Geometry: final body of the model. Coordinates: model frame, mm. Give positions to 0.01 mm unless a question says otherwise; leave off trailing zeros. Write each loop counter-clockwise with the first axis right and the second up, starting at its lowest first coordinate (ties: lowest second). Pieces come first, ordered by that corner, then holes. Notation, with made-up numbers: M -40,-0.75 L -18,-0.75 A17 cw -18,32.25 Z; hole C 56,-3.5 d7. An arc over 180 degrees is marked long. Use a Markdown table: item, result. Add a question column.
(1) Cut plane B-B (y = 326). Output: boundary loops of the cut face in (x, z) (3 decimals), plus the area to 3 significant figures.
(2) Pin query (flat end, axial travel): pin 1 Ø1 at (y, z) = (349.5, 1) entering from +X; pin 2 Ø1.6 at (x, z) = (287, 1.5) entering from +Y; pin 3 Ø1.6 at (x, z) = (287.5, 1.5) entering from -Y. Return the tip coordinate at first contact, or that it passes through.
(3) Cut plane C-C (x = 226.5). Output: boundary loops of the cut face in (y, z) (3 decimals).
(4) Material intervals for L1, parallel to X at y = -335.5, z = 0.75; L2, parallel to Y at x = 267, z = 1.4; L3, parallel to Y at x = 165, z = 1.85, sorted ascending.
(5) Cut plane A-A (z = 1.1). Output: boundary loops of the cut face in (x, y).
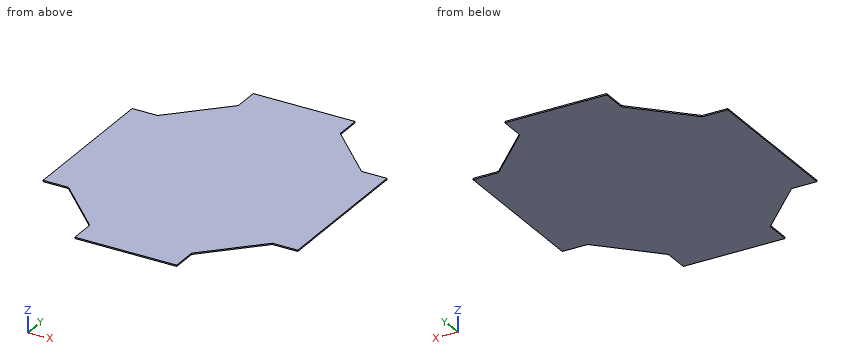
```python
from build123d import *

# Parameters (mm, degrees)
SKETCH1_W           = 635
SKETCH1_H           = 762
BOSS_EXTRUDE1_DEPTH = 3.175
SKETCH3_W           = 901.746898996
SKETCH3_H           = 1073.20581641
CUT_EXTRUDE1_DEPTH  = 496.961017243


with BuildPart() as part:
    # Sketch1 → Boss-Extrude1 (new body)
    with BuildSketch(Plane.XY):
        Rectangle(SKETCH1_W, SKETCH1_H)
    extrude(amount=BOSS_EXTRUDE1_DEPTH)

    # Sketch3 → Cut-Extrude1 (cut, through all)
    with BuildSketch(Plane.XY.offset(3.175)):
        with Locations((-17.044225779, -39.145238765)):
            Rectangle(SKETCH3_W, SKETCH3_H)
        Polygon((-127, 381), (127, 381), (127, 317.5), (254, 190.5), (317.5, 190.5), (317.5, -190.5), (254, -190.5), (127, -317.5), (127, -381), (-127, -381), (-127, -317.5), (-254, -190.5), (-317.5, -190.5), (-317.5, 190.5), (-254, 190.5), (-127, 317.5), align=None, mode=Mode.SUBTRACT)
    extrude(amount=-CUT_EXTRUDE1_DEPTH, mode=Mode.SUBTRACT)


solid = part.part
```
Answer list:
| question | item | result |
|---|---|---|
| 1 | outline | M -127,0 L 127,0 L 127,3.175 L -127,3.175 Z |
| 1 | area | 806 mm² |
| 2 | pin 1 | x = 127 |
| 2 | pin 2 | y = 190.5 |
| 2 | pin 3 | y = -190.5 |
| 3 | outline | M -218,0 L 218,0 L 218,3.175 L -218,3.175 Z |
| 4 | L1 | -127 to 127 |
| 4 | L2 | -190.5 to 190.5 |
| 4 | L3 | -279.5 to 279.5 |
| 5 | outline | M -317.5,-190.5 L -254,-190.5 L -127,-317.5 L -127,-381 L 127,-381 L 127,-317.5 L 254,-190.5 L 317.5,-190.5 L 317.5,190.5 L 254,190.5 L 127,317.5 L 127,381 L -127,381 L -127,317.5 L -254,190.5 L -317.5,190.5 Z |
